from build123d import *

# Parameters (mm, degrees)
SKETCH1_W           = 175
SKETCH1_H           = 51
BOSS_EXTRUDE1_DEPTH = 15
CUT_EXTRUDE3_DEPTH  = 52
SKETCH7_W           = 4.75
SKETCH7_H           = 4.75
CUT_EXTRUDE5_DEPTH  = 145
SKETCH8_W           = 10.05
SKETCH8_H           = 24
CUT_EXTRUDE6_DEPTH  = 16
SKETCH9_W           = 10.05
SKETCH9_H           = 8.05
CUT_EXTRUDE7_DEPTH  = 8


with BuildPart() as part:
    # Sketch1 → Boss-Extrude1 (new body)
    with BuildSketch(Plane(origin=(0, 0, 0), x_dir=(0, 0, -1), z_dir=(1, 0, 0))):
        with Locations((22.937921078, 5.057266603)):
            Rectangle(SKETCH1_W, SKETCH1_H)
    extrude(amount=BOSS_EXTRUDE1_DEPTH)

    # Sketch6 → Cut-Extrude3 (cut, through all)
    with BuildSketch(Plane(origin=(0, 30.557266603, 0), x_dir=(1, 0, 0), z_dir=(0, 1, 0))):
        Polygon((12.5, -60.062078922), (15, -60.062078922), (15, -57.062078922), (12.5, -57.062078922), (5.75, -57.062078922), (5.75, -62.062078922), (12.5, -62.062078922), align=None)
    extrude(amount=-CUT_EXTRUDE3_DEPTH, mode=Mode.SUBTRACT)

    # Sketch7 → Cut-Extrude5 (cut)
    with BuildSketch(Plane(origin=(0, 0, -110.437921078), x_dir=(-1, 0, 0), z_dir=(0, 0, -1))):
        with Locations((-12.625, 0.432266603)):
            Rectangle(SKETCH7_W, SKETCH7_H)
        with Locations((-12.625, 18.432266603)):
            Rectangle(SKETCH7_W, SKETCH7_H)
    extrude(amount=-CUT_EXTRUDE5_DEPTH, mode=Mode.SUBTRACT)

    # Sketch8 → Cut-Extrude6 (cut)
    with BuildSketch(Plane(origin=(0, 0, -110.437921078), x_dir=(-1, 0, 0), z_dir=(0, 0, -1))):
        with Locations((-9.975, 9.557266603)):
            Rectangle(SKETCH8_W, SKETCH8_H)
    extrude(amount=-CUT_EXTRUDE6_DEPTH, mode=Mode.SUBTRACT)

    # Sketch9 → Cut-Extrude7 (cut)
    with BuildSketch(Plane(origin=(0, -2.442733397, 0), x_dir=(1, 0, 0), z_dir=(0, 1, 0))):
        with Locations((9.975, 98.462921078)):
            Rectangle(SKETCH9_W, SKETCH9_H)
    extrude(amount=-CUT_EXTRUDE7_DEPTH, mode=Mode.SUBTRACT)


solid = part.part
Input: part model. Units: mm. Frame: model coordinates. A direction names the side the tool comes from. Coordinates: 2 decimals unless noted, no trailing zeros. Loops run counter-clockwise (first coordinate to the right, second up) from the corner with the lowest first, then second, coordinate; pieces in that order, holes last.
Q1. Set-up query: faces 4 (the face through (10, -6, -102.488)), 5 (the face through (9, 5, 62.062)), 6 (the face through (10, -2.443, -107)), 7 (the face through (15, 5, 62)), 8 (the face through (4, 5, -110.438)). Return all of +Z, -Z, +X, -X, +Y, -Y with unobstructed straight access to the full face (end or side cutting, diameter ignored); none if empty.
Q2. Cut plane C-C (y = 5). Output: boundary loops of the cut face in (x, z), then the cut area to 3 significant figures.
Q3. Cut plane A-A (y = 25.5). Output: boundary loops of the cut face in (x, z).
Q4. Cut plane B-B (z = -33). Output: boundary loops of the cut face in (x, y).
Q5. Contact query for a flat-ended pin moving along its axis: pin 1 (4 mm diameter, centred on x = 13, y = 1, fed in from -Z). Output: stop coordinate, or through.
Q6. Draft query along Y for faces 1 (the face through (7, -20.443, -22)), 2 (the face through (10, 5, 57.062)), 3 (the face through (13, 18, 34.562)). Return one class per face: +Y half, -Y half, draft (parallel to the pull), parting line (faces both ways), or undercut.
Q7. Material intervals for line 1 (Y direction, x = 14.25, z = 15); line 2 (Z direction, x = 9.75, y = -4.5); line 3 (Z direction, x = 8.5, y = -11.5), sorted ascending.
Working result:
1. face 4: +X
1. face 5: +Y, -Y
1. face 6: -Z, +X
1. face 7: +Z, -Z, +X, +Y, -Y
1. face 8: -Z, +X, -X, +Y, -Y
2. outline: (0, -110.44) - (4.95, -110.44) - (4.95, -94.44) - (15, -94.44) - (15, 57.06) - (5.75, 57.06) - (5.75, 62.06) - (12.5, 62.06) - (12.5, 60.06) - (15, 60.06) - (15, 64.56) - (0, 64.56) - close
2. area: 2,420 mm2
3. outline: (0, -110.44) - (15, -110.44) - (15, 57.06) - (5.75, 57.06) - (5.75, 62.06) - (12.5, 62.06) - (12.5, 60.06) - (15, 60.06) - (15, 64.56) - (0, 64.56) - close
4. outline: (0, -20.44) - (15, -20.44) - (15, -1.94) - (10.25, -1.94) - (10.25, 2.81) - (15, 2.81) - (15, 16.06) - (10.25, 16.06) - (10.25, 20.81) - (15, 20.81) - (15, 30.56) - (0, 30.56) - close
5. pin 1: stops at z = -94.44
6. face 1: -Y half
6. face 2: draft
6. face 3: undercut
7. line 1: y = -20.44 to -1.94, 2.81 to 16.06, 20.81 to 30.56
7. line 2: z = -110.44 to -102.49, -94.44 to 57.06, 62.06 to 64.56
7. line 3: z = -110.44 to 57.06, 62.06 to 64.56
